The listing builds one solid part. Answer for the finished solid, in the listing's coordinates (mm). A direction names the side the tool comes from. Give positions to 0.01 mm unless a question says otherwise; leave off trailing zeros. Write each loop counter-clockwise with the first axis right and the second up, starting at its lowest first coordinate (ties: lowest second). Pieces come first, ordered by that corner, then holes. Notation, with made-up numbers: (-11.75, 18.25) -> (-1.75, 18.25) arc R12 cw to (-1.75, 22.25) -> close; hole circle Ø6 at (61, 37.5). An arc over 180 degrees is marked (long way). Put each result on its own line as item: value. Start each with the question number.
1) A cutting plane is placed at A-A (y = -1). Write down the section's boundary in (x, z).
2) Flat-ended cylindrical pins translate along their axes: pin 1 Ø2 at (y, z) = (-12, 1.5) entering from -X; pin 2 Ø1 at (y, z) = (11, 1.5) entering from -X. Find the tip coordinate at first contact, or state that the pin passes through.
3) A cutting plane is placed at B-B (x = -11). Write down the section's boundary in (y, z), then the cut area to 3 significant figures.
4) A cutting plane is placed at C-C (z = 2.6). Give the number of separate pieces and of enclosed holes in the cut face, then the cut area to 3 significant figures.
5) Find the intervals of material crossed by line 1 along Y through (x, z) = (-39, 3.55); line 2 along Y through (x, z) = (48.5, 3.45); line 3 along Y through (x, z) = (7, 0.5), in increasing order. Write a range as from..to.
6) For a pull along X with two mould halves and no side action, classify faces 1 (the flat face through (2, -4, 4)), 2 (the flat face through (54.253, -12.811, 1.972)), 3 (the cylindrical face through (2.003, 0.631, 1.972)), 4 (the flat face through (-30, 10, 2)) as released by +X, released by -X, zero draft, split by the parting line, or undercut.
7) A cutting plane is placed at D-D (x = 24.5). Write down the section's boundary in (y, z), then the cut area to 3 significant figures.
8) For faces 5 (the cylindrical face through (-6.615, -0.566, 1.972)), 6 (the flat face through (-18.639, -10.645, 2.028)), 7 (the cylindrical face through (-23.65, 12.01, 1.97)), determine the directions among +Z, -Z, +X, -X, +Y, -Y from which every point of the face is accessible in a straight line to the end or side of a thin tool.
from build123d import *

# Parameters (mm, degrees)
SKETCH_1_R          = 2.1
EXTRUDE_1_DEPTH     = 4
FILLET_3_R          = 5
CUT_EXTRUDE_1_DEPTH = 48.602520942
SKETCH_5_R          = 1.6
CUT_EXTRUDE_4_DEPTH = 45.060309279
SKETCH_6_R          = 2.6
EXTRUDE_3_DEPTH     = 4
FILLET_4_R          = 3
EXTRUDE_6_DEPTH     = 4
SKETCH_8_R          = 1.6
CUT_EXTRUDE_5_DEPTH = 59.484887667
CUT_EXTRUDE_6_DEPTH = 59.484887667
SKETCH_10_R         = 1.6
EXTRUDE_5_DEPTH     = 4
CUT_EXTRUDE_7_DEPTH = 59.131742072
FILLET_5_R          = 3
SKETCH_13_R         = 2.6
CUT_EXTRUDE_8_DEPTH = 10
SKETCH_14_R         = 1.6
CUT_EXTRUDE_9_DEPTH = 10


with BuildPart() as part:
    # 草图1 → 凸台-拉伸1 (new body)
    with BuildSketch(Plane.XY):
        with BuildLine():
            Line((-30, 15), (-30, 8))
            Line((-30, 8), (-3.625760775, -6.565352908))
            ThreePointArc((-3.625760775, -6.565352908), (-2.508336586, -7.068114853), (-1.323960706, -7.382217014))
            Line((-1.323960706, -7.382217014), (30, -13))
            Line((30, -13), (40, -13))
            ThreePointArc((40, -13), (44.961129361, -8.622250323), (41.234825739, -3.154878186))
            Line((41.234825739, -3.154878186), (-8.89090638, 9.620145142))
            Line((-8.89090638, 9.620145142), (-30, 15))
        make_face()
        Circle(SKETCH_1_R, mode=Mode.SUBTRACT)
    extrude(amount=EXTRUDE_1_DEPTH)

    # 圆角3
    fillet_3_edges = [part.edges().sort_by_distance(p)[0] for p in [
        (30, -13, 2),
    ]]
    fillet(fillet_3_edges, radius=FILLET_3_R)

    # 草图2 → 切除-拉伸1 (cut, through all)
    with BuildSketch(Plane.XY.offset(4)):
        Polygon((41.234825739, -3.154878186), (38.343573198, -14.499370217), (44.079449635, -18.425378343), (50.650422799, -6.675561263), (42.473370603, -0.777871599), align=None)
    extrude(amount=-CUT_EXTRUDE_1_DEPTH, mode=Mode.SUBTRACT)

    # 草图5 → 切除-拉伸4 (cut, through all)
    with BuildSketch(Plane.XY.offset(4)):
        with Locations((-27, 10.5)):
            Circle(SKETCH_5_R)
        with BuildLine():
            Line((-27, 13.75), (-27.802461724, 17.848471623))
            Line((-27.802461724, 17.848471623), (-34.200130402, 16.595837785))
            Line((-34.200130402, 16.595837785), (-34.200130402, 10.5))
            Line((-34.200130402, 10.5), (-30.25, 10.5))
            ThreePointArc((-30.25, 10.5), (-29.298097039, 12.798097039), (-27, 13.75))
        make_face()
    extrude(amount=-CUT_EXTRUDE_4_DEPTH, mode=Mode.SUBTRACT)

    # 草图6 → 凸台-拉伸3 (add)
    with BuildSketch(Plane.XY.offset(4)):
        with BuildLine():
            Line((-1.323960706, -7.382217014), (-35.888817872, -13.896208466))
            ThreePointArc((-35.888817872, -13.896208466), (-42.336413013, -10.742753389), (-41.147636408, -3.664436343))
            Line((-41.147636408, -3.664436343), (-30, 7))
            Line((-30, 7), (-30, 8))
            Line((-30, 8), (-1.323960706, -7.382217014))
        make_face()
        with Locations((-37, -8)):
            Circle(SKETCH_6_R, mode=Mode.SUBTRACT)
    extrude(amount=-EXTRUDE_3_DEPTH)

    # 圆角4
    fillet_4_edges = [part.edges().sort_by_distance(p)[0] for p in [
        (41.234825739, -3.154878186, 2),
        (-1.323960706, -7.382217014, 2),
        (38.725702071, -13, 2),
        (-30, 7, 2),
    ]]
    fillet(fillet_4_edges, radius=FILLET_4_R)

    # 草图12 → 凸台-拉伸6 (add, through all)
    with BuildSketch(Plane(origin=(0, 0, 0), x_dir=(-1, 0, 0), z_dir=(0, 0, -1))):
        Polygon((-38.32775265, -2.413982742), (-55.770191182, -6.859355403), (-53.147184729, -17.151322425), (-28.912835061, -12.805022846), align=None)
    extrude(amount=-EXTRUDE_6_DEPTH)

    # 草图8 → 切除-拉伸5 (cut, through all)
    with BuildSketch(Plane(origin=(0, 0, 0), x_dir=(-1, 0, 0), z_dir=(0, 0, -1))):
        with Locations((-18.803711615, -5.177837216)):
            Circle(SKETCH_8_R)
        with Locations((-28.493955243, -7.647488694)):
            Circle(SKETCH_8_R)
        with Locations((-38.184198872, -10.117140172)):
            Circle(SKETCH_8_R)
    extrude(amount=-CUT_EXTRUDE_5_DEPTH, mode=Mode.SUBTRACT)

    # 草图9 → 切除-拉伸6 (cut, through all)
    with BuildSketch(Plane(origin=(0, 0, 0), x_dir=(-1, 0, 0), z_dir=(0, 0, -1))):
        with BuildLine():
            Line((30, 11.75), (30, 25.879948008))
            Line((30, 25.879948008), (-59.978637955, 25.879948008))
            Line((-59.978637955, 25.879948008), (-59.978637955, -9.479867102))
            Line((-59.978637955, -9.479867102), (22.437617221, 11.52470556))
            ThreePointArc((22.437617221, 11.52470556), (23.662682687, 12.016789899), (24.71625119, 12.812356238))
            ThreePointArc((24.71625119, 12.812356238), (27.640627923, 13.686235375), (30, 11.75))
        make_face()
    extrude(amount=-CUT_EXTRUDE_6_DEPTH, mode=Mode.SUBTRACT)

    # 草图10 → 凸台-拉伸5 (add, through all)
    with BuildSketch(Plane(origin=(0, 0, 0), x_dir=(-1, 0, 0), z_dir=(0, 0, -1))):
        with BuildLine():
            Line((30, 11.75), (30, 9.25))
            ThreePointArc((30, 9.25), (23.75, 10.5), (30, 11.75))
        make_face()
        with Locations(Location((27, 10.5, 0), (0, 0, 180))):
            Circle(SKETCH_10_R, mode=Mode.SUBTRACT)
    extrude(amount=-EXTRUDE_5_DEPTH)

    # 草图11 → 切除-拉伸7 (cut, through all)
    with BuildSketch(Plane(origin=(0, 0, 0), x_dir=(-1, 0, 0), z_dir=(0, 0, -1))):
        with BuildLine():
            Line((24.825037002, 5.031136033), (29.169175717, 0.875296258))
            ThreePointArc((29.169175717, 0.875296258), (30.06075817, -4.433441527), (25.225061815, -6.798532835))
            Line((25.225061815, -6.798532835), (9.462787836, -3.82802098))
            ThreePointArc((9.462787836, -3.82802098), (6.612728883, -0.499278448), (9.246599393, 3.003019229))
            Line((9.246599393, 3.003019229), (21.072085472, 6.016857713))
            ThreePointArc((21.072085472, 6.016857713), (23.076090116, 6.009539302), (24.825037002, 5.031136033))
        make_face()
    extrude(amount=-CUT_EXTRUDE_7_DEPTH, mode=Mode.SUBTRACT)

    # 圆角5
    fillet_5_edges = [part.edges().sort_by_distance(p)[0] for p in [
        (53.147184729, -17.151322425, 2),
        (55.39974346, -8.312891947, 2),
    ]]
    fillet(fillet_5_edges, radius=FILLET_5_R)

    # 草图13 → 切除-拉伸8 (cut)
    with BuildSketch(Plane(origin=(0, 0, 0), x_dir=(-1, 0, 0), z_dir=(0, 0, -1))):
        with Locations((-48.605919829, -11.741249861)):
            Circle(SKETCH_13_R)
    extrude(amount=-CUT_EXTRUDE_8_DEPTH, mode=Mode.SUBTRACT)

    # 草图14 → 切除-拉伸9 (cut)
    with BuildSketch(Plane.XY.offset(4)):
        with Locations((-24.257929074, -9.024692947)):
            Circle(SKETCH_14_R)
    extrude(amount=-CUT_EXTRUDE_9_DEPTH, mode=Mode.SUBTRACT)


solid = part.part
Reply:
1. outline: (-38.36, 0) -> (-30.34, 0) -> (-30.34, 4) -> (-38.36, 4) -> close; (-6.66, 0) -> (-1.85, 0) -> (-1.85, 4) -> (-6.66, 4) -> close; (1.85, 0) -> (26.71, 0) -> (26.71, 4) -> (1.85, 4) -> close
2. pin 1: stops at x = -42.2
2. pin 2: stops at x = -30
3. outline: (-9.21, 0) -> (-4.12, 0) -> (-4.12, 4) -> (-9.21, 4) -> close; (3.45, 0) -> (8.61, 0) -> (8.61, 4) -> (3.45, 4) -> close
3. area: 41.0 mm2
4. separate pieces: 1
4. enclosed holes: 9
4. area: 1,070 mm2
5. line 1: y = -13.66..-9.66, -6.34..-1.61
5. line 2: y = -16.32..-14.34, -9.14..-6.55
5. line 3: y = -8.88..4.02
6. face 1: zero draft
6. face 2: released by +X
6. face 3: undercut
6. face 4: released by -X
7. outline: (-12.01, 0) -> (-0.44, 0) -> (-0.44, 4) -> (-12.01, 4) -> close
7. area: 46.3 mm2
8. face 5: +Z, -Z
8. face 6: +Z, -Z, -Y
8. face 7: +Z, -Z, +X, +Y
